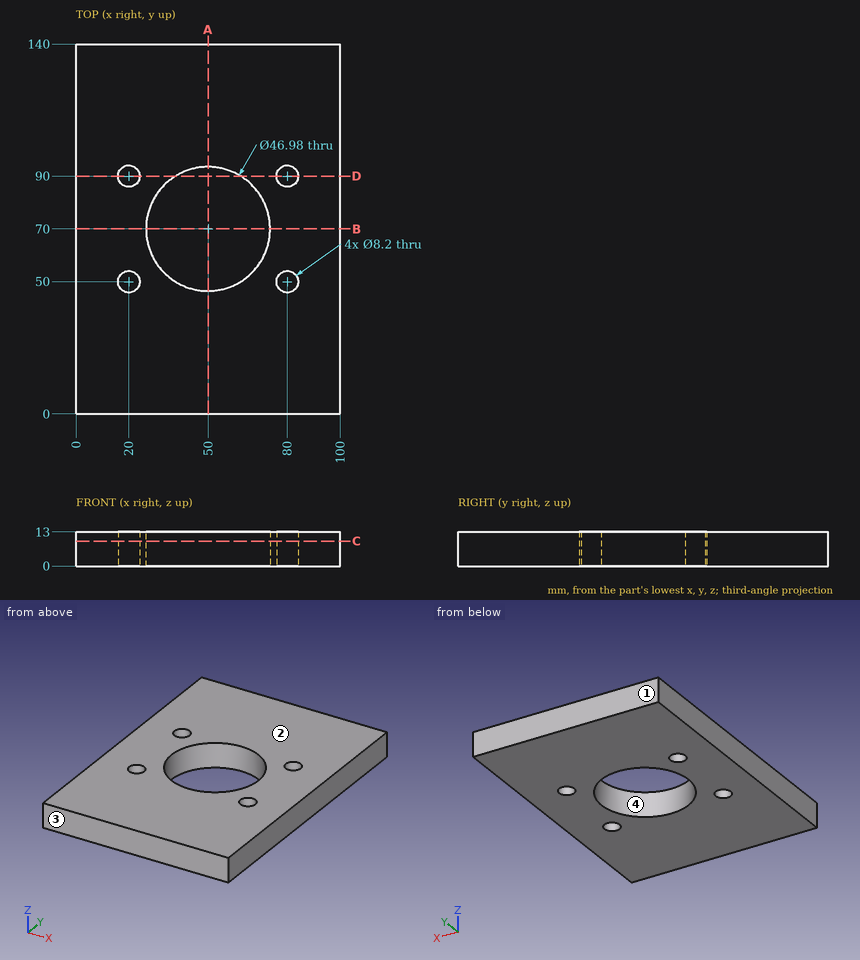
Source: three-view drawing plus pictorial views. Frame: mm from the lowest corner of the part. Round coordinates to 2 decimals unless told otherwise and drop trailing zeros. Write each loop counter-clockwise with the first axis right and the second up, starting at its lowest first coordinate (ties: lowest second). Pieces come first, ordered by that corner, then holes. Notation, with made-up numbers: M -11,62 L -6,62 A28 cw -6,94 Z; hole C 84.5,-25 d1. An arc over 180 degrees is marked long. Write item = value, one per line.
Item 1: Material intervals for line 1 along Y through (x, z) = (80, 10.25); line 2 along Y through (x, z) = (50, 8.75); line 3 along X through (y, z) = (70, 8), sorted ascending. Write a range as [from, to].
Findings:
line_1 = [0, 45.9], [54.1, 85.9], [94.1, 140]
line_2 = [0, 46.51], [93.49, 140]
line_3 = [0, 26.51], [73.49, 100]
Item 2: Section query D-D on y = 90. Return loops of the section in (x, z).
Findings:
outline = M 0,0 L 15.9,0 L 15.9,13 L 0,13 Z; M 24.1,0 L 37.68,0 L 37.68,13 L 24.1,13 Z; M 62.32,0 L 75.9,0 L 75.9,13 L 62.32,13 Z; M 84.1,0 L 100,0 L 100,13 L 84.1,13 Z
Item 3: Section query B-B on y = 70. Return loops of the section in (x, z), then the cut area to 3 significant figures.
Findings:
outline = M 0,0 L 26.51,0 L 26.51,13 L 0,13 Z; M 73.49,0 L 100,0 L 100,13 L 73.49,13 Z
area = 689 mm^2
Item 4: Pin query (flat end, axial travel): P1, Ø5, axis at x = 33, z = 1.5, coming from the -Y side; P2, Ø5, axis at x = 20, y = 50, coming from the +Z side. Return the tip coordinate at first contact, or that it passes through.
Findings:
P1 = 0
P2 = through
Item 5: Section query A-A on x = 50. Return loops of the section in (y, z), then the cut area to 3 significant figures.
Findings:
outline = M 0,0 L 46.51,0 L 46.51,13 L 0,13 Z; M 93.49,0 L 140,0 L 140,13 L 93.49,13 Z
area = 1,210 mm^2
Item 6: Section query C-C on z = 9.5. Return loops of the section in (x, y), then the cut area to 3 significant figures.
Findings:
outline = M 0,0 L 100,0 L 100,140 L 0,140 Z; hole C 20,50 d8.2; hole C 20,90 d8.2; hole C 50,70 d46.98; hole C 80,50 d8.2; hole C 80,90 d8.2
area = 12,100 mm^2
Item 7: Pull-direction query (Y, two-part tool) for the marked faces 1, 2, 3 and 4; classes: pulls with the +Y half, pulls with the -Y half, needs draft (parallel to the pull), parting line crosses it, or undercut.
Findings:
face_1 = pulls with the +Y half
face_2 = needs draft
face_3 = pulls with the -Y half
face_4 = undercut
